from build123d import *

# Parameters (mm, degrees)
SKETCH1_R          = 89
SKETCH1_R_2        = 66.5
SKETCH1_R_3        = 5.25
BASE_FLANGE1_DEPTH = 0.7366


# Sheet-metal steps are written as plain solids
with BuildPart() as part:
    # Sketch1 → Base-Flange1 (new body)
    with BuildSketch(Plane(origin=(0, 0, 0), x_dir=(1, 0, 0), z_dir=(0, 1, 0))):
        with Locations(Location((0, 0, 0), (0, 0, 270))):
            Circle(SKETCH1_R)
        with Locations(Location((0, 0, 0), (0, 0, 270))):
            Circle(SKETCH1_R_2, mode=Mode.SUBTRACT)
        with Locations(Location((26.677571179, 73.296024421, 0), (0, 0, 270))):
            Circle(SKETCH1_R_3, mode=Mode.SUBTRACT)
        with Locations(Location((-26.677571179, 73.296024421, 0), (0, 0, 270))):
            Circle(SKETCH1_R_3, mode=Mode.SUBTRACT)
        with Locations(Location((-76.815004735, 13.544557858, 0), (0, 0, 270))):
            Circle(SKETCH1_R_3, mode=Mode.SUBTRACT)
        with Locations(Location((-76.815004735, -13.544557858, 0), (0, 0, 270))):
            Circle(SKETCH1_R_3, mode=Mode.SUBTRACT)
        with Locations(Location((-26.677571179, -73.296024421, 0), (0, 0, 270))):
            Circle(SKETCH1_R_3, mode=Mode.SUBTRACT)
        with Locations(Location((26.677571179, -73.296024421, 0), (0, 0, 270))):
            Circle(SKETCH1_R_3, mode=Mode.SUBTRACT)
        with Locations(Location((76.815004735, 13.544557858, 0), (0, 0, 270))):
            Circle(SKETCH1_R_3, mode=Mode.SUBTRACT)
        with Locations(Location((76.815004735, -13.544557858, 0), (0, 0, 270))):
            Circle(SKETCH1_R_3, mode=Mode.SUBTRACT)
    extrude(amount=-BASE_FLANGE1_DEPTH)


solid = part.part
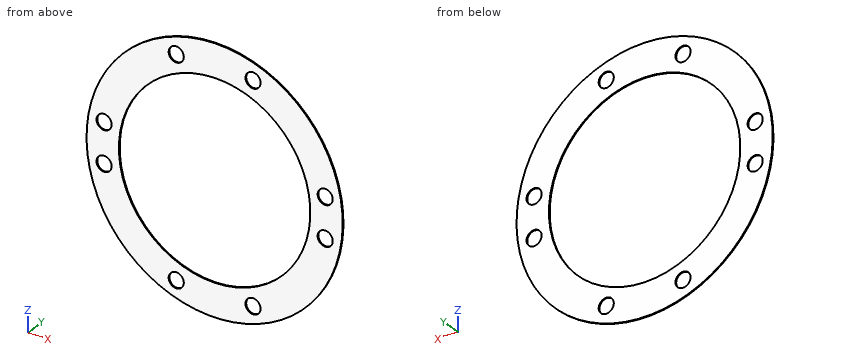
Read the model definition and answer for the solid it produces. Units are mm, in the model's axes. Give positions to 0.01 mm unless a question says otherwise; leave off trailing zeros. Write each loop counter-clockwise with the first axis right and the second up, starting at its lowest first coordinate (ties: lowest second). Pieces come first, ordered by that corner, then holes. Notation, with made-up numbers: M 0,-32 L 27,-32 A8 ccw 27,-18 Z; hole C 46.25,-12 d11. An arc over 180 degrees is marked long. One line per item, written item: value. Start each with the question number.
(1) Find section B-B (z = 0). Determine the outline of the cut face in (x, y).
(2) Find the intervals of material crossed by line 1 (Z direction, x = 80.5, y = -0.7); line 2 (Z direction, x = -74, y = -0.3); line 3 (X direction, y = -0.5, z = -12), in increasing order.
(3) Find section A-A (x = 0). Determine the outline of the cut face in (y, z), plus the area to 3 significant figures.
(4) Find section C-C (y = -0.15). Give the number of separate pieces and of enclosed holes in the cut face, plus the area to 3 significant figures.
(5) A flat-ended cylindrical pin translates along its axis: pin 1 Ø17 at (x, z) = (-76.82, 13.54) entering from -Y. Find the tip coordinate at first contact, or state that the pin passes through.
Results below:
1. outline: M -89,-0.74 L -66.5,-0.74 L -66.5,0 L -89,0 Z; M 66.5,-0.74 L 89,-0.74 L 89,0 L 66.5,0 Z
2. line 1: z = -37.96 to -17.28, -9.81 to 9.81, 17.28 to 37.96
2. line 2: z = -49.45 to -17.98, -9.11 to 9.11, 17.98 to 49.45
2. line 3: x = -88.19 to -81.83, -71.8 to -65.41, 65.41 to 71.8, 81.83 to 88.19
3. outline: M -0.74,-89 L 0,-89 L 0,-66.5 L -0.74,-66.5 Z; M -0.74,66.5 L 0,66.5 L 0,89 L -0.74,89 Z
3. area: 33.1 mm^2
4. separate pieces: 1
4. enclosed holes: 9
4. area: 10,300 mm^2
5. pin 1: stops at y = -0.74
